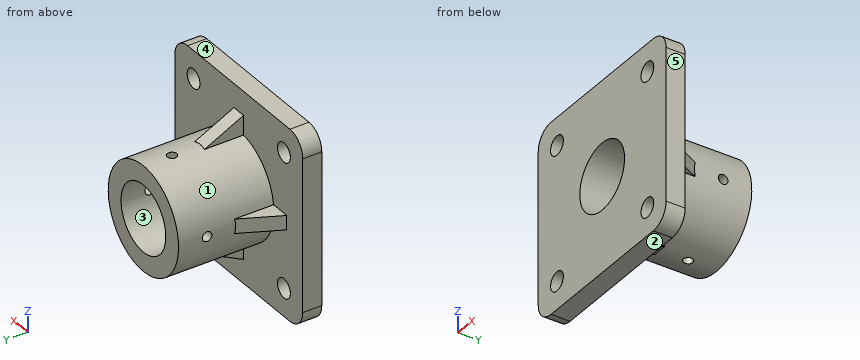
```python
from build123d import *

# Parameters (mm, degrees)
SKETCH2_R           = 10
SKETCH2_R_2         = 35
BOSS_EXTRUDE1_DEPTH = 20
SKETCH5_R           = 55
SKETCH5_R_2         = 35
BOSS_EXTRUDE2_DEPTH = 100
RIB1_REACH          = 187.472
SKETCH6_WALL_W      = 417.66609937
SKETCH6_WALL_H      = 15
CIRPATTERN1_COUNT   = 4
SKETCH7_R           = 5
CUT_EXTRUDE2_DEPTH  = 186.47236991
CIRPATTERN2_COUNT   = 4


with BuildPart() as part:
    # Sketch2 → Boss-Extrude1 (new body)
    with BuildSketch(Plane(origin=(0, 0, 0), x_dir=(1, 0, 0), z_dir=(0, 1, 0))):
        with BuildLine():
            Line((-80, -100), (80, -100))
            ThreePointArc((80, -100), (94.142135624, -94.142135624), (100, -80))
            Line((100, -80), (100, 80))
            ThreePointArc((100, 80), (94.142135624, 94.142135624), (80, 100))
            Line((80, 100), (-80, 100))
            ThreePointArc((-80, 100), (-94.142135624, 94.142135624), (-100, 80))
            Line((-100, 80), (-100, -80))
            ThreePointArc((-100, -80), (-94.142135624, -94.142135624), (-80, -100))
        make_face()
        with Locations(Location((-70.710678119, 70.710678119, 0), (0, 0, 270))):
            Circle(SKETCH2_R, mode=Mode.SUBTRACT)
        with Locations(Location((70.710678119, 70.710678119, 0), (0, 0, 270))):
            Circle(SKETCH2_R, mode=Mode.SUBTRACT)
        with Locations(Location((-70.710678119, -70.710678119, 0), (0, 0, 270))):
            Circle(SKETCH2_R, mode=Mode.SUBTRACT)
        with Locations(Location((70.710678119, -70.710678119, 0), (0, 0, 270))):
            Circle(SKETCH2_R, mode=Mode.SUBTRACT)
        with Locations(Location((0, 0, 0), (0, 0, 270))):
            Circle(SKETCH2_R_2, mode=Mode.SUBTRACT)
    extrude(amount=BOSS_EXTRUDE1_DEPTH)

    # Sketch5 → Boss-Extrude2 (add)
    with BuildSketch(Plane(origin=(0, 20, 0), x_dir=(1, 0, 0), z_dir=(0, 1, 0))):
        with Locations(Location((0, 0, 0), (0, 0, 90))):
            Circle(SKETCH5_R)
        with Locations(Location((0, 0, 0), (0, 0, 270))):
            Circle(SKETCH5_R_2, mode=Mode.SUBTRACT)
    extrude(amount=BOSS_EXTRUDE2_DEPTH)

    # Sketch6 wall → Rib1 (add, up to next)
    with BuildSketch(Plane(origin=(65, 40, 0), x_dir=(0.4472135955, -0.894427191, 0), z_dir=(0.894427191, 0.4472135955, 0)), mode=Mode.PRIVATE) as rib1_sk1:
        Rectangle(SKETCH6_WALL_W, SKETCH6_WALL_H)
    rib1_tool1 = extrude(rib1_sk1.sketch, amount=-RIB1_REACH, mode=Mode.PRIVATE) - part.part
    rib1 = rib1_tool1.solids().sort_by_distance((65, 40, 0))[0]
    add(rib1)

    # CirPattern1: Rib1 ×4 about axis
    cirpattern1_axis = Axis((0, 0, 0), (0, 1, 0))
    for i in range(1, CIRPATTERN1_COUNT):
        add(rib1.rotate(cirpattern1_axis, i * 360 / CIRPATTERN1_COUNT))

    # Sketch7 → Cut-Extrude2 (cut, through all)
    with BuildSketch(Plane.XY):
        with Locations(Location((0, 90, 0), (0, 0, 90))):
            Circle(SKETCH7_R)
    cut_extrude2 = extrude(amount=-CUT_EXTRUDE2_DEPTH, mode=Mode.SUBTRACT)

    # CirPattern2: Cut-Extrude2 ×4 about axis
    cirpattern2_axis = Axis((0, 0, 0), (0, -1, 0))
    for i in range(1, CIRPATTERN2_COUNT):
        add(cut_extrude2.rotate(cirpattern2_axis, i * 360 / CIRPATTERN2_COUNT), mode=Mode.SUBTRACT)


solid = part.part
```
Could you check a few things on this model? Use its own coordinates, in mm. Face numbers are marked on the shaded views. A direction names the side the tool comes from. Coordinates: 2 decimals unless noted, no trailing zeros. Write each loop counter-clockwise with the first axis right and the second up, starting at its lowest first coordinate (ties: lowest second). Pieces come first, ordered by that corner, then holes. Notation, with made-up numbers: (-11, 19.25) -> (4, 19.25) arc R13 cw to (4, 41.25) -> close; hole circle Ø9 at (80, 22). An arc over 180 degrees is marked (long way). Return JSON: item names as keys, results as strings.
(1) Imagine slicing it at C-C, the plane y = 26. Please give me the cut outline in (x, z).
Numbers:
{"outline": "(-72, -7.5) -> (-54.49, -7.5) arc R55 ccw to (-7.5, -54.49) -> (-7.5, -72) -> (7.5, -72) -> (7.5, -54.49) arc R55 ccw to (54.49, -7.5) -> (72, -7.5) -> (72, 7.5) -> (54.49, 7.5) arc R55 ccw to (7.5, 54.49) -> (7.5, 72) -> (-7.5, 72) -> (-7.5, 54.49) arc R55 ccw to (-54.49, 7.5) -> (-72, 7.5) -> close; hole circle Ø70 at (0, 0)"}
(2) I'm going to push flat-ended pins straight in: pin 1 (6 mm diameter, centred on x = -50.5, z = -43, fed in from -Y); pin 2 (6 mm diameter, centred on y = 90, z = 0, fed in from -X); pin 3 (1 mm diameter, centred on x = 26, y = 51, fed in from -Z); pin 4 (22.5 mm diameter, centred on y = 39, z = -59.5, fed in from -X). Where does each tip first touch, or does it pass through?
Numbers:
{"pin 1": "stops at y = 0", "pin 2": "passes through", "pin 3": "stops at z = -48.73", "pin 4": "stops at x = -26.4"}
(3) Imagine slicing it at A-A, the plane z = 0. Please give me the cut outline in (x, y).
Numbers:
{"outline": "(-100, 0) -> (-35, 0) -> (-35, 85) -> (-55, 85) -> (-55, 60) -> (-75, 20) -> (-100, 20) -> close; (-55, 95) -> (-35, 95) -> (-35, 120) -> (-55, 120) -> close; (35, 0) -> (100, 0) -> (100, 20) -> (75, 20) -> (55, 60) -> (55, 85) -> (35, 85) -> close; (35, 95) -> (55, 95) -> (55, 120) -> (35, 120) -> close"}
(4) I need wall thicknesses on L1, parallel to Y at x = 50.75, z = 0; L2, parallel to Z at x = 39, y = 90; L3, parallel to Y at x = 38.5, z = 81.5. Which ranges of each line are inside material? Lowest first, please.
Numbers:
{"L1": "y = 0 to 85, 95 to 120", "L2": "z = -38.78 to -5, 5 to 38.78", "L3": "y = 0 to 20"}
(5) Which directions (+Z, -Z, +X, -X, +Y, -Y) give clear straight access to the entire face, cutting with the end or side of a thin tool? Please do the marked faces 1 and 2.
Numbers:
{"face 1": "+Y", "face 2": "-Z, +X, -X, +Y, -Y"}
(6) Imagine slicing it at D-D, the plane z = 64.5. Please give me the cut outline in (x, y), then the cut area to 3 significant figures.
Numbers:
{"outline": "(-100, 0) -> (-78.55, 0) -> (-78.55, 20) -> (-100, 20) -> close; (-62.87, 0) -> (62.87, 0) -> (62.87, 20) -> (7.5, 20) -> (7.5, 41) -> (-7.5, 41) -> (-7.5, 20) -> (-62.87, 20) -> close; (78.55, 0) -> (100, 0) -> (100, 20) -> (78.55, 20) -> close", "area": "3,690 mm2"}
(7) We'd pull the mould along Z, two halves only. Please class the marked faces 3, 4 and 5: +Z half, -Z half, draft (parallel to the pull), parting line (faces both ways), or undercut.
Numbers:
{"face 3": "undercut", "face 4": "+Z half", "face 5": "draft"}
(8) Imagine slicing it at B-B, the plane x = -23.5. Please give me the cut outline in (y, z).
Numbers:
{"outline": "(0, -100) -> (20, -100) -> (20, -49.73) -> (120, -49.73) -> (120, -25.94) -> (0, -25.94) -> close; (0, 25.94) -> (120, 25.94) -> (120, 49.73) -> (20, 49.73) -> (20, 100) -> (0, 100) -> close"}
